```python
from build123d import *

# Parameters (mm, degrees)
SKETCH1_R       = 16.3068
FEATURE_A_DEPTH = 101.6
SKETCH2_W       = 32.6136
SKETCH2_H       = 12.7
FEATURE_B_DEPTH = 25.908
SKETCH3_W       = 63.3984
SKETCH3_H       = 25.4
FEATURE_C_DEPTH = 25.4
SKETCH4_W       = 25.4
SKETCH4_H       = 63.4746
FEATURE_D_DEPTH = 25.3746
SKETCH5_W       = 50.75428
SKETCH5_H       = 25.4
FEATURE_E_DEPTH = 25.4


with BuildPart() as part:
    # Sketch1 → Feature A (new body)
    with BuildSketch(Plane.XY):
        Circle(SKETCH1_R)
    extrude(amount=FEATURE_A_DEPTH)

    # Sketch2 → Feature B (add)
    with BuildSketch(Plane(origin=(0, 0, 0), x_dir=(1, 0, 0), z_dir=(0, 1, 0))):
        with Locations((0, -6.35)):
            Rectangle(SKETCH2_W, SKETCH2_H)
    extrude(amount=FEATURE_B_DEPTH)

    # Sketch3 → Feature C (add)
    with BuildSketch(Plane(origin=(0, 25.908, 0), x_dir=(1, 0, 0), z_dir=(0, 1, 0))):
        with Locations((0, -12.7)):
            Rectangle(SKETCH3_W, SKETCH3_H)
    feature_c = extrude(amount=FEATURE_C_DEPTH)

    # Sketch4 → Feature D (add)
    with BuildSketch(Plane(origin=(31.6992, 0, 0), x_dir=(0, 0, -1), z_dir=(1, 0, 0))):
        with Locations((-12.7, 57.6453)):
            Rectangle(SKETCH4_W, SKETCH4_H)
    feature_d = extrude(amount=FEATURE_D_DEPTH)

    # Sketch5 → Feature E (add)
    with BuildSketch(Plane(origin=(0, 89.3826, 0), x_dir=(1, 0, 0), z_dir=(0, 1, 0))):
        with Locations((31.69666, -12.7)):
            Rectangle(SKETCH5_W, SKETCH5_H)
    feature_e = extrude(amount=FEATURE_E_DEPTH)

    # Mirror6: Feature C, Feature D, Feature E across plane
    add(feature_c.mirror(Plane.ZY))
    add(feature_d.mirror(Plane.ZY))
    add(feature_e.mirror(Plane.ZY))


solid = part.part
```
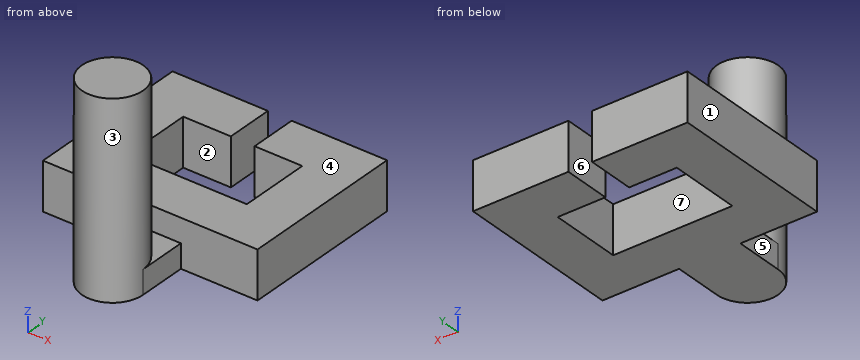
Read the model definition and answer for the solid it produces. Units are mm, in the model's axes. Face numbers are marked on the shaded views. A direction names the side the tool comes from. Coordinates: 2 decimals unless noted, no trailing zeros. Loops run counter-clockwise (first coordinate to the right, second up) from the corner with the lowest first, then second, coordinate; pieces in that order, holes last.
(1) The mould has two halves that part along X. Classify the marked faces 1, 2 and 3: released by +X, released by -X, zero draft, split by the parting line, or undercut.
Solution:
face 1: released by -X
face 2: undercut
face 3: split by the parting line
(2) The part is cut by section C-C (x = -30). Determine the outline of the cut face in (y, z).
Solution:
outline: (25.91, 0) - (51.31, 0) - (51.31, 25.4) - (25.91, 25.4) - close; (89.38, 0) - (114.78, 0) - (114.78, 25.4) - (89.38, 25.4) - close
(3) The part is cut by section A-A (y = 62). Determine the outline of the cut face in (x, z).
Solution:
outline: (-57.07, 0) - (-31.7, 0) - (-31.7, 25.4) - (-57.07, 25.4) - close; (31.7, 0) - (57.07, 0) - (57.07, 25.4) - (31.7, 25.4) - close
(4) A tool of negligible diameter and unlimited length cuts with its end or side. For the marked faces 4, 5, 6 and 7, from which of +Z, -Z, +X, -X, +Y, -Y can it reach the whole face along a straight path? Write none if from no direction.
Solution:
face 4: +Z, +X, -X, +Y
face 5: +Z, -Z, -X, -Y
face 6: +Z, -Z, +Y
face 7: +Z, -Z
(5) Flat-ended cylindrical pins translate along their axes: pin 1 Ø5 at (x, z) = (8.5, 63) entering from -Y; pin 2 Ø6 at (x, z) = (-5.5, 89) entering from +Y; pin 3 Ø4 at (x, z) = (-1.5, 25) entering from +Y. Find the tip coordinate at first contact, or state that the pin passes through.
Solution:
pin 1: stops at y = -15.16
pin 2: stops at y = 16.11
pin 3: stops at y = 51.31
(6) Consider line 1 along Y through (x, z) = (-30.5, 20.5); line 2 along X through (y, z) = (93.5, 9.5); line 3 along Z through (x, y) = (3, 29). Determine where each line is inside the solid, lowest interval first.
Solution:
line 1: y = 25.91 to 51.31, 89.38 to 114.78
line 2: x = -57.07 to -6.32, 6.32 to 57.07
line 3: z = 0 to 25.4
(7) The part is cut by section D-D (x = 0). Determine the outline of the cut face in (y, z).
Solution:
outline: (-16.31, 0) - (51.31, 0) - (51.31, 25.4) - (25.91, 25.4) - (25.91, 12.7) - (16.31, 12.7) - (16.31, 101.6) - (-16.31, 101.6) - close
(8) The part is cut by section B-B (z = 14.5). Determine the outline of the cut face in (x, y).
Solution:
outline: (-57.07, 25.91) - (57.07, 25.91) - (57.07, 114.78) - (6.32, 114.78) - (6.32, 89.38) - (31.7, 89.38) - (31.7, 51.31) - (-31.7, 51.31) - (-31.7, 89.38) - (-6.32, 89.38) - (-6.32, 114.78) - (-57.07, 114.78) - close; circle Ø32.61 at (0, 0)
